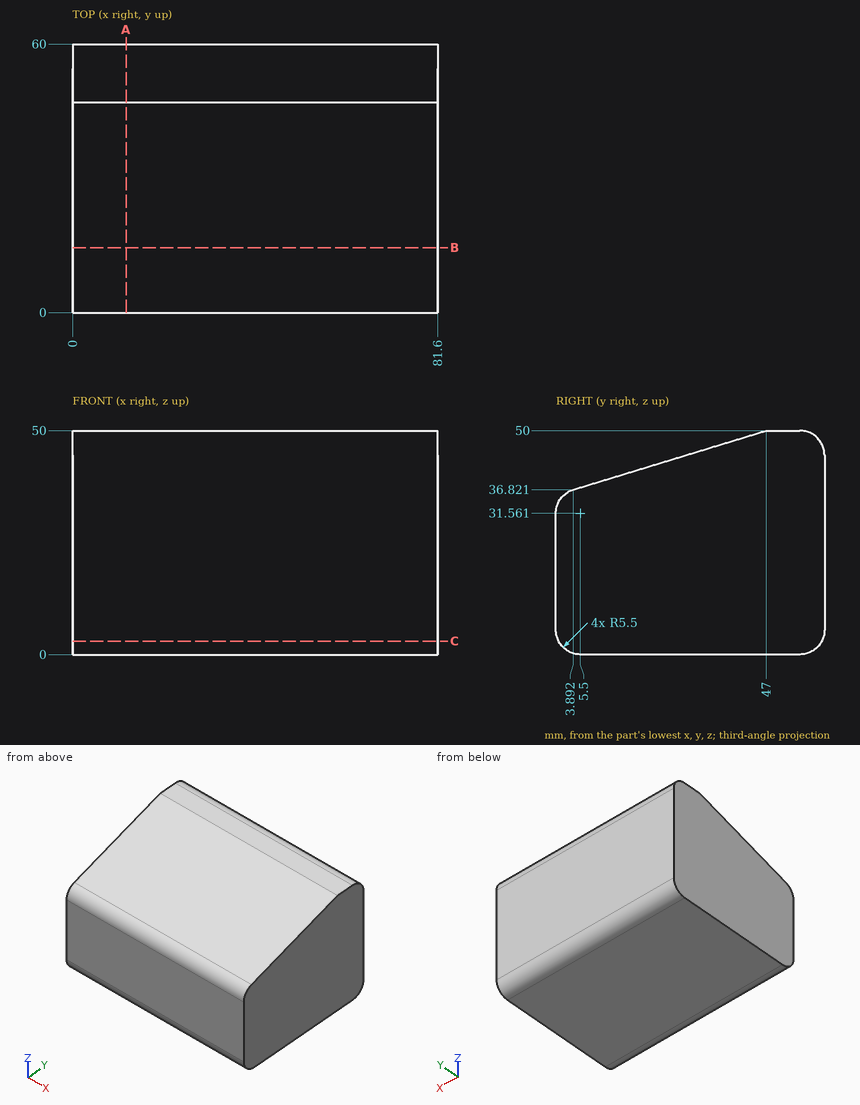
Geometry check sheet. Reference: drawing and pictorial views, mm from the part's lowest x, y, z. Round coordinates to 2 decimals unless told otherwise and drop trailing zeros. Order: outer loops, then holes, each group sorted by start corner. A loop starts at its lowest first (then second) coordinate and runs counter-clockwise, first axis right, second up. Notation, with made-up numbers: (21.25, 57.5) - (47.25, 57.5) arc R15 ccw to (47.25, 86.5) - close; hole circle Ø8 at (-27.5, 81). An arc over 180 degrees is marked (long way). One line per question, with ' | ' between items. Start each with the question number.
(1) Sectioned sample at B-B on y = 14.5. Record the cut outline in (x, z), and give its area (3 significant figures).
(2) Depth check by flat-ended pin: pin 1 Ø5 at (x, y) = (64, 27.5) entering from +Z. Enter the tip coordinate at first touch or a pass-through.
(3) Thickness scan on L1, parallel to Y at x = 18.5, z = 32; L2, parallel to Z at x = 51.5, y = 55; L3, parallel to Z at x = 31.5, y = 32 (1 decimal). Record the ranges inside material, lowest first. Write a range as [from, to].
(4) Sectioned sample at A-A on x = 12. Record the cut outline in (y, z), and give its area (3 significant figures).
(5) Sectioned sample at C-C on z = 3. Record the cut outline in (x, y).
Conclusion:
1) outline: (0, 0) - (81.6, 0) - (81.6, 40.06) - (0, 40.06) - close | area: 3,270 mm2
2) pin 1: stops at z = 44.8
3) L1: y = [0.02, 60] | L2: z = [0.02, 49.98] | L3: z = [0, 45.4]
4) outline: (0, 5.5) arc R5.5 ccw to (5.5, 0) - (54.5, 0) arc R5.5 ccw to (60, 5.5) - (60, 44.5) arc R5.5 ccw to (54.5, 50) - (47, 50) - (3.89, 36.82) arc R5.5 ccw to (0, 31.56) - close | area: 2,640 mm2
5) outline: (0, 0.6) - (81.6, 0.6) - (81.6, 59.4) - (0, 59.4) - close
